Input: part model. Units: mm. Frame: model coordinates. A direction names the side the tool comes from. Round coordinates to 2 decimals unless told otherwise and drop trailing zeros. Loops run counter-clockwise (first coordinate to the right, second up) from the corner with the lowest first, then second, coordinate; pieces in that order, holes last. Notation, with made-up numbers: (69.5, 0.5) -> (78.5, 0.5) arc R24 ccw to (78.5, 22.5) -> close; hole circle Ø9 at (34.25, -40). An arc over 180 degrees is marked (long way). Answer as a JSON object with one key per item and string values. Group by question number.
Item 1: Section query C-C on x = 5.5. Return loops of the section in (y, z).
Item 2: Section query A-A on y = 3.25. Return loops of the section in (x, z), and give its area (3 significant figures).
Item 3: Pin query (flat end, axial travel): pin 1 (5 mm diameter, centred on x = 2.5, y = 5.5, fed in from +Z). Return the tip coordinate at first contact, or that it passes through.
Item 4: Draft query along X for faces 1 (the flat face through (-4.1, 2.7, 4.9)), 2 (the flat face through (0, 4.45, 5)), 3 (the flat face through (0, -8.25, 5)), 4 (the flat face through (8.25, 0, 5)). Return one class per face: released by +X, released by -X, zero draft, split by the parting line, or undercut.
Item 5: Set-up query: faces 5 (the flat face through (0.6, 2.5, 0)), 6 (the flat face through (-5.063, -4.497, 4.93)). Return all of +Z, -Z, +X, -X, +Y, -Y with unobstructed straight access to the full face (end or side cutting, diameter ignored); none if empty.
Item 6: Section query B-B on z = 1.5. Return loops of the section in (x, y), and give its area (3 significant figures).
Item 7: Material intervals for line 1 (Y direction, x = 0, z = 7); line 2 (X direction, y = -1, z = 2); line 3 (Y direction, x = 1.5, z = 2.25), sorted ascending. Write a range as [from, to].
Item 8: Section query D-D on y = -0.75. Return loops of the section in (x, z).
from build123d import *

# Parameters (mm, degrees)
F0_W     = 16.5
F0_H     = 16.5
F1_DEPTH = 10


# Not quite as in the source:
# - a feature names something its author has since deleted; it is built from what else it names


with BuildPart() as f1:
    # F0 (on Top) → F1 (new body)
    with BuildSketch(Plane.XY):
        Rectangle(F0_W, F0_H)
        Polygon((6.8843145751, 7.45), (7.45, 7.45), (7.45, 6.8843145751), (7.45, -6.8843145751), (7.45, -7.45), (6.8843145751, -7.45), (-6.8843145751, -7.45), (-7.45, -7.45), (-7.45, -6.8843145751), (-7.45, 6.8843145751), (-7.45, 7.45), (-6.8843145751, 7.45), (-5.05, 7.45), (-4.25, 7.45), (4.25, 7.45), (5.05, 7.45), align=None, mode=Mode.SUBTRACT)
        Polygon((-4.25, 4.8156854249), (-4.25, 7.45), (-5.05, 7.45), (-5.05, 5.6156854249), align=None)
        Polygon((-4.25, 4.45), (-4.25, 4.8156854249), (-5.05, 5.6156854249), (-5.05, 4.4843145751), (-4.2156854249, 3.65), (-3.0843145751, 3.65), (-3.8843145751, 4.45), align=None)
        Polygon((7.45, 6.8843145751), (7.45, 7.45), (6.8843145751, 7.45), (5.05, 5.6156854249), (5.05, 4.4843145751), align=None)
        Polygon((-5.05, 5.6156854249), (-6.8843145751, 7.45), (-7.45, 7.45), (-7.45, 6.8843145751), (-5.05, 4.4843145751), align=None)
        with BuildLine():
            Line((-1.2828041187, 1.8484895437), (-2.1758154582, 2.7415008831))
            ThreePointArc((-2.1758154582, 2.7415008831), (-2.4748737342, 2.4748737342), (-2.7415008831, 2.1758154582))
            Line((-2.7415008831, 2.1758154582), (-1.8484895437, 1.2828041187))
            ThreePointArc((-1.8484895437, 1.2828041187), (-1.5909902577, 1.5909902577), (-1.2828041187, 1.8484895437))
        make_face()
        with BuildLine():
            ThreePointArc((-3.0738154941, 1.6738154941), (-3.4870317978, -0.3010136893), (-2.7415008831, -2.1758154582))
            Line((-2.7415008831, -2.1758154582), (-1.8484895437, -1.2828041187))
            ThreePointArc((-1.8484895437, -1.2828041187), (-2.25, 0), (-1.8484895437, 1.2828041187))
            Line((-1.8484895437, 1.2828041187), (-2.7415008831, 2.1758154582))
            ThreePointArc((-2.7415008831, 2.1758154582), (-2.9184717118, 1.9319738268), (-3.0738154941, 1.6738154941))
        make_face()
        with BuildLine():
            ThreePointArc((-2.7415008831, -2.1758154582), (-2.4748737342, -2.4748737342), (-2.1758154582, -2.7415008831))
            Line((-2.1758154582, -2.7415008831), (-1.2828041187, -1.8484895437))
            ThreePointArc((-1.2828041187, -1.8484895437), (-1.5909902577, -1.5909902577), (-1.8484895437, -1.2828041187))
            Line((-1.8484895437, -1.2828041187), (-2.7415008831, -2.1758154582))
        make_face()
        with BuildLine():
            Line((-7.45, -7.45), (-6.8843145751, -7.45))
            Line((-6.8843145751, -7.45), (-2.1758154582, -2.7415008831))
            ThreePointArc((-2.1758154582, -2.7415008831), (-2.4748737342, -2.4748737342), (-2.7415008831, -2.1758154582))
            Line((-2.7415008831, -2.1758154582), (-7.45, -6.8843145751))
            Line((-7.45, -6.8843145751), (-7.45, -7.45))
        make_face()
        with BuildLine():
            ThreePointArc((-2.1758154582, -2.7415008831), (0, -3.5), (2.1758154582, -2.7415008831))
            Line((2.1758154582, -2.7415008831), (1.2828041187, -1.8484895437))
            ThreePointArc((1.2828041187, -1.8484895437), (0, -2.25), (-1.2828041187, -1.8484895437))
            Line((-1.2828041187, -1.8484895437), (-2.1758154582, -2.7415008831))
        make_face()
        with BuildLine():
            ThreePointArc((2.1758154582, -2.7415008831), (2.4748737342, -2.4748737342), (2.7415008831, -2.1758154582))
            Line((2.7415008831, -2.1758154582), (1.8484895437, -1.2828041187))
            ThreePointArc((1.8484895437, -1.2828041187), (1.5909902577, -1.5909902577), (1.2828041187, -1.8484895437))
            Line((1.2828041187, -1.8484895437), (2.1758154582, -2.7415008831))
        make_face()
        with BuildLine():
            Line((1.8484895437, -1.2828041187), (2.7415008831, -2.1758154582))
            ThreePointArc((2.7415008831, -2.1758154582), (3.3049397189, -1.1521169448), (3.5, 0))
            ThreePointArc((3.5, 0), (3.3917808176, 0.8636103782), (3.0738154941, 1.6738154941))
            ThreePointArc((3.0738154941, 1.6738154941), (2.9184717118, 1.9319738268), (2.7415008831, 2.1758154582))
            Line((2.7415008831, 2.1758154582), (1.8484895437, 1.2828041187))
            ThreePointArc((1.8484895437, 1.2828041187), (2.1472775174, 0.672085756), (2.25, 0))
            ThreePointArc((2.25, 0), (2.1472775174, -0.672085756), (1.8484895437, -1.2828041187))
        make_face()
        with BuildLine():
            Line((7.45, -7.45), (7.45, -6.8843145751))
            Line((7.45, -6.8843145751), (2.7415008831, -2.1758154582))
            ThreePointArc((2.7415008831, -2.1758154582), (2.4748737342, -2.4748737342), (2.1758154582, -2.7415008831))
            Line((2.1758154582, -2.7415008831), (6.8843145751, -7.45))
            Line((6.8843145751, -7.45), (7.45, -7.45))
        make_face()
        with BuildLine():
            Line((1.8484895437, 1.2828041187), (2.7415008831, 2.1758154582))
            ThreePointArc((2.7415008831, 2.1758154582), (2.4748737342, 2.4748737342), (2.1758154582, 2.7415008831))
            Line((2.1758154582, 2.7415008831), (1.2828041187, 1.8484895437))
            ThreePointArc((1.2828041187, 1.8484895437), (1.5909902577, 1.5909902577), (1.8484895437, 1.2828041187))
        make_face()
        Polygon((5.05, 4.4843145751), (5.05, 5.6156854249), (4.25, 4.8156854249), (4.25, 4.45), (3.8843145751, 4.45), (3.0843145751, 3.65), (4.2156854249, 3.65), align=None)
        Polygon((5.05, 3.65), (5.05, 4.4843145751), (4.2156854249, 3.65), align=None)
        Polygon((5.05, 5.6156854249), (5.05, 7.45), (4.25, 7.45), (4.25, 4.8156854249), align=None)
        Polygon((3.0843145751, 3.65), (3.8843145751, 4.45), (-3.8843145751, 4.45), (-3.0843145751, 3.65), align=None)
        Polygon((5.05, 5.6156854249), (6.8843145751, 7.45), (5.05, 7.45), align=None)
        Polygon((-5.05, 5.6156854249), (-5.05, 7.45), (-6.8843145751, 7.45), align=None)
        Polygon((-5.05, 3.65), (-4.2156854249, 3.65), (-5.05, 4.4843145751), align=None)
        with BuildLine():
            Line((2.1758154582, 2.7415008831), (3.0843145751, 3.65))
            Line((3.0843145751, 3.65), (-3.0843145751, 3.65))
            Line((-3.0843145751, 3.65), (-2.1758154582, 2.7415008831))
            ThreePointArc((-2.1758154582, 2.7415008831), (0, 3.5), (2.1758154582, 2.7415008831))
        make_face()
        with BuildLine():
            Line((-2.1758154582, 2.7415008831), (-3.0843145751, 3.65))
            Line((-3.0843145751, 3.65), (-4.2156854249, 3.65))
            Line((-4.2156854249, 3.65), (-2.7415008831, 2.1758154582))
            ThreePointArc((-2.7415008831, 2.1758154582), (-2.4748737342, 2.4748737342), (-2.1758154582, 2.7415008831))
        make_face()
        with BuildLine():
            Line((2.7415008831, 2.1758154582), (4.2156854249, 3.65))
            Line((4.2156854249, 3.65), (3.0843145751, 3.65))
            Line((3.0843145751, 3.65), (2.1758154582, 2.7415008831))
            ThreePointArc((2.1758154582, 2.7415008831), (2.4748737342, 2.4748737342), (2.7415008831, 2.1758154582))
        make_face()
        with BuildLine():
            Line((-2.7415008831, 2.1758154582), (-4.2156854249, 3.65))
            Line((-4.2156854249, 3.65), (-5.05, 3.65))
            Line((-5.05, 3.65), (-3.0738154941, 1.6738154941))
            ThreePointArc((-3.0738154941, 1.6738154941), (-2.9184717118, 1.9319738268), (-2.7415008831, 2.1758154582))
        make_face()
        with BuildLine():
            Line((3.0738154941, 1.6738154941), (5.05, 3.65))
            Line((5.05, 3.65), (4.2156854249, 3.65))
            Line((4.2156854249, 3.65), (2.7415008831, 2.1758154582))
            ThreePointArc((2.7415008831, 2.1758154582), (2.9184717118, 1.9319738268), (3.0738154941, 1.6738154941))
        make_face()
        with BuildLine():
            Line((1.2828041187, 1.8484895437), (2.1758154582, 2.7415008831))
            ThreePointArc((2.1758154582, 2.7415008831), (0, 3.5), (-2.1758154582, 2.7415008831))
            Line((-2.1758154582, 2.7415008831), (-1.2828041187, 1.8484895437))
            ThreePointArc((-1.2828041187, 1.8484895437), (0, 2.25), (1.2828041187, 1.8484895437))
        make_face()
    extrude(amount=F1_DEPTH)


solid = f1.part
Solved:
{
 "1": {"outline": "(-8.25, 0) -> (-7.45, 0) -> (-7.45, 10) -> (-8.25, 10) -> close; (-6.07, 0) -> (-4.93, 0) -> (-4.93, 10) -> (-6.07, 10) -> close; (4.93, 0) -> (8.25, 0) -> (8.25, 10) -> (4.93, 10) -> close"},
 "2": {"outline": "(-8.25, 0) -> (-7.45, 0) -> (-7.45, 10) -> (-8.25, 10) -> close; (-4.65, 0) -> (4.65, 0) -> (4.65, 10) -> (-4.65, 10) -> close; (7.45, 0) -> (8.25, 0) -> (8.25, 10) -> (7.45, 10) -> close", "area": "109 mm²"},
 "3": {"pin 1": "z = 10"},
 "4": {"face 1": "undercut", "face 2": "undercut", "face 3": "zero draft", "face 4": "released by +X"},
 "5": {"face 5": "-Z, +X, -X, +Y, -Y", "face 6": "+Z, -Z"},
 "6": {"outline": "(-8.25, -8.25) -> (8.25, -8.25) -> (8.25, 8.25) -> (-8.25, 8.25) -> close; hole (-7.45, -6.88) -> (-2.74, -2.18) arc R3.5 cw to (-3.07, 1.67) -> (-5.05, 3.65) -> (-5.05, 4.48) -> (-7.45, 6.88) -> close; hole (-6.88, -7.45) -> (6.88, -7.45) -> (2.18, -2.74) arc R3.5 cw to (-2.18, -2.74) -> close; hole (-4.25, 4.45) -> (4.25, 4.45) -> (4.25, 7.45) -> (-4.25, 7.45) -> close; hole circle Ø4.5 at (0, 0); hole (2.74, -2.18) -> (7.45, -6.88) -> (7.45, 6.88) -> (5.05, 4.48) -> (5.05, 3.65) -> (3.07, 1.67) arc R3.5 cw to start", "area": "113 mm²"},
 "7": {"line 1": "[-8.25, -7.45], [-3.5, -2.25], [2.25, 4.45], [7.45, 8.25]", "line 2": "[-8.25, -7.45], [-3.35, -2.02], [2.02, 3.35], [7.45, 8.25]", "line 3": "[-8.25, -7.45], [-3.16, -1.68], [1.68, 4.45], [7.45, 8.25]"},
 "8": {"outline": "(-8.25, 0) -> (-7.45, 0) -> (-7.45, 10) -> (-8.25, 10) -> close; (-3.42, 0) -> (-2.12, 0) -> (-2.12, 10) -> (-3.42, 10) -> close; (2.12, 0) -> (3.42, 0) -> (3.42, 10) -> (2.12, 10) -> close; (7.45, 0) -> (8.25, 0) -> (8.25, 10) -> (7.45, 10) -> close"}
}
